Can you work these out from the model? Positions are in its coordinate system, mm. A direction names the side the tool comes from. Round coordinates to 2 decimals unless told otherwise and drop trailing zeros. Loops run counter-clockwise (first coordinate to the right, second up) from the corner with the lowest first, then second, coordinate; pieces in that order, holes last. Notation, with made-up numbers: (-20.75, -3.5) - (25.25, -3.5) arc R29 ccw to (25.25, 24.5) - close; hole circle Ø7 at (41, -37.75). An arc over 180 degrees is marked (long way). Answer as CSV lines item,"result".
```python
from build123d import *

# Parameters (mm, degrees)
SKETCH1_R               = 9.75
BOSS_EXTRUDE1_DEPTH     = 45
SKETCH2_R               = 11.75
BOSS_EXTRUDE2_DEPTH     = 3
CUT_EXTRUDE1_DEPTH      = 13
CUT_EXTRUDE1_DEPTH_BACK = 23
CUT_EXTRUDE2_DEPTH      = 23
CUT_EXTRUDE2_DEPTH_BACK = 23
SKETCH5_R               = 1.5


with BuildPart() as part:
    # Sketch1 → Boss-Extrude1 (new body)
    with BuildSketch(Plane.XY):
        with Locations(Location((0, 0, 0), (0, 0, 180))):
            Circle(SKETCH1_R)
    extrude(amount=BOSS_EXTRUDE1_DEPTH)

    # Sketch2 → Boss-Extrude2 (add)
    with BuildSketch(Plane.XY.offset(45)):
        Circle(SKETCH2_R)
    extrude(amount=BOSS_EXTRUDE2_DEPTH)

    # Sketch4 → Cut-Extrude1 (cut, two sides: drawn at the far end of the back side and taken through both)
    with BuildSketch(Plane(origin=(0, 0, 0), x_dir=(1, 0, 0), z_dir=(0, 1, 0)).offset(-CUT_EXTRUDE1_DEPTH_BACK)):
        with BuildLine():
            Line((2.80710702, -12.735), (2.80710702, -35.735))
            ThreePointArc((2.80710702, -35.735), (0, -38.54210702), (-2.80710702, -35.735))
            Line((-2.80710702, -35.735), (-2.80710702, -12.735))
            ThreePointArc((-2.80710702, -12.735), (0, -9.92789298), (2.80710702, -12.735))
        make_face()
    extrude(amount=CUT_EXTRUDE1_DEPTH + CUT_EXTRUDE1_DEPTH_BACK, mode=Mode.SUBTRACT)

    # Sketch5 → Cut-Extrude2 (cut, two sides: drawn at the far end of the back side and taken through both)
    with BuildSketch(Plane(origin=(0, 0, 0), x_dir=(1, 0, 0), z_dir=(0, 1, 0)).offset(-CUT_EXTRUDE2_DEPTH_BACK)):
        with Locations(Location((0, -3.556649542, 0), (0, 0, 90))):
            Circle(SKETCH5_R)
    extrude(amount=CUT_EXTRUDE2_DEPTH + CUT_EXTRUDE2_DEPTH_BACK, mode=Mode.SUBTRACT)


solid = part.part
```
Q1. Imagine slicing it at A-A (y = 0). Write out the boundary of the cut face in (x, z) (3 decimals), then the cut area to 3 significant figures.
Checks:
outline,"(-11.75, 45) - (-9.75, 45) - (-9.75, 0) - (9.75, 0) - (9.75, 45) - (11.75, 45) - (11.75, 48) - (-11.75, 48) - close; hole (-2.807, 12.735) arc R2.807 ccw to (2.807, 12.735) - (2.807, 35.735) arc R2.807 ccw to (-2.807, 35.735) - close; hole circle Ø3 at (0, 3.557)"
area,"787 mm²"
Q2. We'd pull the mould along X, two halves only. Please class faces 3 (the flat face through (2, 10, 45)), 4 (the flat face through (-2.807, 0, 24)), 5 (the cylindrical face through (-9.3, -2.93, 22.18)): pulls with the +X half, pulls with the -X half, needs draft (parallel to the pull), parting line crosses it, or undercut.
Checks:
face 3,"needs draft"
face 4,"undercut"
face 5,"parting line crosses it"
Q3. On a 3-axis mill with a long thin cutter (end or side, diameter ignored), from which of +Z, -Z, +X, -X, +Y, -Y can I reach the whole of each face in a straight line? I mean faces 1 (the cylindrical face through (0.06, -0.14, 38.54)), 2 (the flat face through (0, 0, 48)). Say none if no direction works.
Checks:
face 1,"+Y, -Y"
face 2,"+Z, +X, -X, +Y, -Y"
Q4. I'm going to push flat-ended pins straight in: pin 1 Ø1 at (x, z) = (9.5, 42.5) entering from -Y; pin 2 Ø5.5 at (y, z) = (-2, 19) entering from -X; pin 3 Ø1.5 at (y, z) = (-9, 39) entering from -X. Where does each tip first touch, or does it pass through?
Checks:
pin 1,"y = -3.75"
pin 2,"x = -9.75"
pin 3,"x = -5.2"
Q5. If I drill on line 1 along Z through (x, y) = (0.5, 5); line 2 along X through (y, z) = (-0.25, 41); line 3 along X through (y, z) = (2, 20), over which ranges is the centre line in solid material (lowest first)? Write a range as [from, to].
Checks:
line 1,"[0, 2.14], [4.97, 9.97], [38.5, 48]"
line 2,"[-9.75, 9.75]"
line 3,"[-9.54, -2.81], [2.81, 9.54]"
Q6. Imagine slicing it at C-C (z = 25). Write out the boundary of the cut face in (x, y).
Checks:
outline,"(-2.81, -9.34) - (-2.81, 9.34) arc R9.75 ccw to start; (2.81, -9.34) arc R9.75 ccw to (2.81, 9.34) - close"
Q7. Imagine slicing it at B-B (x = 0). Write out the boundary of the cut face in (y, z).
Checks:
outline,"(-11.75, 45) - (-9.75, 45) - (-9.75, 38.54) - (9.75, 38.54) - (9.75, 45) - (11.75, 45) - (11.75, 48) - (-11.75, 48) - close; (-9.75, 0) - (9.75, 0) - (9.75, 2.06) - (-9.75, 2.06) - close; (-9.75, 5.06) - (9.75, 5.06) - (9.75, 9.93) - (-9.75, 9.93) - close"
Q8. Imagine slicing it at D-D (x = 7). Write out the boundary of the cut face in (y, z), then the cut area to 3 significant figures.
Checks:
outline,"(-9.44, 45) - (-6.79, 45) - (-6.79, 0) - (6.79, 0) - (6.79, 45) - (9.44, 45) - (9.44, 48) - (-9.44, 48) - close"
area,"667 mm²"
